Work out the finished part from the listing and answer in its coordinate system (mm). Face numbers are marked on the shaded views. A direction names the side the tool comes from. Give positions to 0.01 mm unless a question says otherwise; leave off trailing zeros. Write each loop counter-clockwise with the first axis right and the second up, starting at its lowest first coordinate (ties: lowest second). Pieces come first, ordered by that corner, then holes. Notation, with made-up numbers: (48.5, 5) - (87.5, 5) arc R16 ccw to (87.5, 27) - close; hole circle Ø3 at (61, 36.5). An arc over 180 degrees is marked (long way). Write item = value, one per line.
from build123d import *

# Parameters (mm, degrees)
SKETCH_1_R          = 9
EXTRUDE_1_DEPTH     = 1
SKETCH_2_R          = 1.3
CUT_EXTRUDE_1_DEPTH = 2
SKETCH_4_W          = 7.6
SKETCH_4_H          = 2.9
CUT_EXTRUDE_6_DEPTH = 2
SKETCH_5_W          = 1
SKETCH_5_H          = 2
SKETCH_5_W_2        = 2
SKETCH_5_H_2        = 1
EXTRUDE_3_DEPTH     = 9


with BuildPart() as part:
    # ｽｹｯﾁ1 → ﾎﾞｽ - 押し出し1 (new body)
    with BuildSketch(Plane.XY):
        Circle(SKETCH_1_R)
    extrude(amount=EXTRUDE_1_DEPTH)

    # ｽｹｯﾁ2 → ｶｯﾄ - 押し出し1 (cut, through all)
    with BuildSketch(Plane.XY):
        with Locations((0, 6.25)):
            Circle(SKETCH_2_R)
        with Locations((0, -6.25)):
            Circle(SKETCH_2_R)
    extrude(amount=CUT_EXTRUDE_1_DEPTH, mode=Mode.SUBTRACT)

    # ｽｹｯﾁ4 → ｶｯﾄ - 押し出し6 (cut, through all)
    with BuildSketch(Plane.XY):
        with Locations((2.8, 0)):
            Rectangle(SKETCH_4_W, SKETCH_4_H)
    extrude(amount=CUT_EXTRUDE_6_DEPTH, mode=Mode.SUBTRACT)

    # ｽｹｯﾁ5 → ﾎﾞｽ - 押し出し3 (add)
    with BuildSketch(Plane.XY):
        Polygon((-6.363961031, 4.949747468), (-4.949747468, 6.363961031), (-5.656854249, 7.071067812), (-7.071067812, 5.656854249), align=None)
        with Locations((-8.5, 0)):
            Rectangle(SKETCH_5_W, SKETCH_5_H)
        with Locations((0, 8.5)):
            Rectangle(SKETCH_5_W_2, SKETCH_5_H_2)
        Polygon((4.949747468, 6.363961031), (6.363961031, 4.949747468), (7.071067812, 5.656854249), (5.656854249, 7.071067812), align=None)
        with Locations((8.5, 0)):
            Rectangle(SKETCH_5_W, SKETCH_5_H)
        Polygon((6.363961031, -4.949747468), (4.949747468, -6.363961031), (5.656854249, -7.071067812), (7.071067812, -5.656854249), align=None)
        with Locations((0, -8.5)):
            Rectangle(SKETCH_5_W_2, SKETCH_5_H_2)
        Polygon((-4.949747468, -6.363961031), (-6.363961031, -4.949747468), (-7.071067812, -5.656854249), (-5.656854249, -7.071067812), align=None)
    extrude(amount=EXTRUDE_3_DEPTH)


solid = part.part
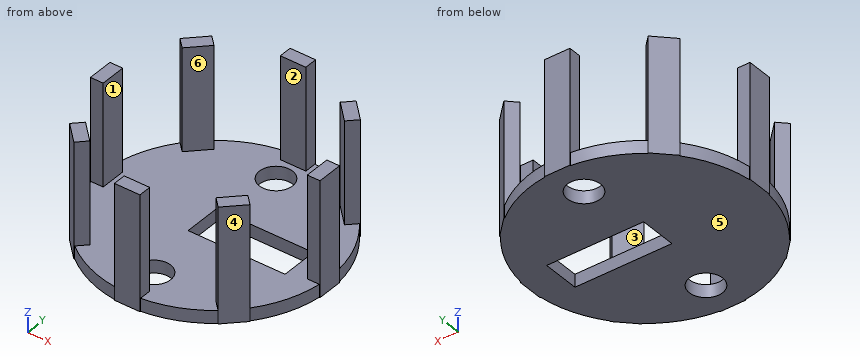
1. Find section D-D, the plane y = -2.75. Give the vertices of the cut face in (x, z), then the cut area to 3 significant figures.
Solution:
outline = (-8.57, 0) - (8.57, 0) - (8.57, 1) - (-8.57, 1) - close
area = 17.1 mm^2
2. Straight lines are drawn through the part: line 1 (Z direction, x = 5.25, y = 6.75); line 2 (X direction, y = -6.25, z = 0.6); line 3 (X direction, y = -5.5, z = 7.75). For each, find the intervals that lie inside material, in ascending order.
Solution:
line_1 = 0 to 1
line_2 = -6.48 to -1.3, 1.3 to 6.48
line_3 = -6.91 to -5.81, 5.81 to 6.91
3. Find section B-B, the plane z = 2.5. Give the number of separate pieces and of enclosed holes in the cut face, then the cut area to 3 significant figures.
Solution:
separate_pieces = 8
enclosed_holes = 0
area = 16.0 mm^2
4. For a pull along Y with two mould halves and no side action, classify the marked faces 4, 5 and 6 as pulls with the +Y half, pulls with the -Y half, needs draft (parallel to the pull), parting line crosses it, or undercut.
Solution:
face_4 = pulls with the -Y half
face_5 = needs draft
face_6 = undercut
5. A tool of negligible diameter and unlimited length cuts with its end or side. For the marked faces 1, 2 and 3, from which of +Z, -Z, +X, -X, +Y, -Y can it reach the whole face along a straight path? Write none if from no direction.
Solution:
face_1 = +Z, +Y, -Y
face_2 = +Z, +X, -X
face_3 = +Z
6. Given pin 1 (0.8 mm diameter, centred on x = 2, z = 0.5, fed in from -Y); pin 2 (3 mm diameter, centred on x = 1.5, y = 6.5, fed in from +Z); pin 3 (8 mm diameter, centred on x = -4, y = 4, fed in from +Z); pin 4 (0.5 mm diameter, centred on x = 8.5, z = 5, fed in from +Y), each flat-ended and moving along its own axis, determine where each tip first touches the part or whether it passes through.
Solution:
pin_1 = -8.86
pin_2 = 1
pin_3 = 9
pin_4 = 1
7. Find section A-A, the plane x = 0. Give the vertices of the cut face in (y, z).
Solution:
outline = (-9, 0) - (-7.55, 0) - (-7.55, 1) - (-8, 1) - (-8, 9) - (-9, 9) - close; (-4.95, 0) - (-1.45, 0) - (-1.45, 1) - (-4.95, 1) - close; (1.45, 0) - (4.95, 0) - (4.95, 1) - (1.45, 1) - close; (7.55, 0) - (9, 0) - (9, 9) - (8, 9) - (8, 1) - (7.55, 1) - close
